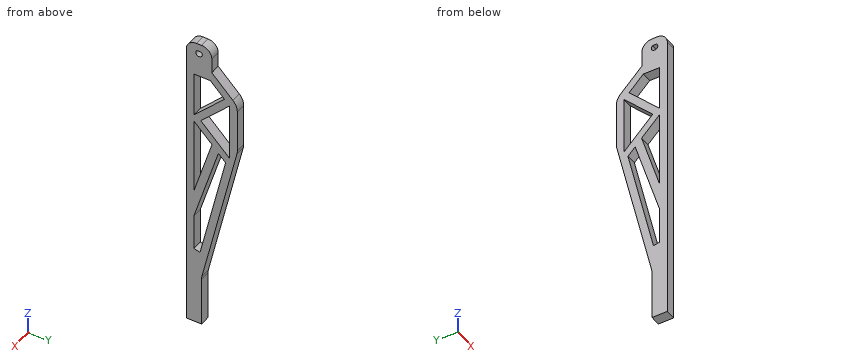
from build123d import *

# Parameters (mm, degrees)
BOSS_EXTRUDE1_DEPTH = 10
CUT_EXTRUDE2_DEPTH  = 305.302481094
FILLET1_R           = 10
FILLET2_R           = 15


with BuildPart() as part:
    # Sketch1 → Boss-Extrude1 (new body)
    with BuildSketch(Plane(origin=(0, 0, 0), x_dir=(0, 0, -1), z_dir=(1, 0, 0))):
        Polygon((0, 0), (300, 0), (300, 15), (250, 15), (100, 50), (50, 50), (25, 25), (0, 25), align=None)
    extrude(amount=-BOSS_EXTRUDE1_DEPTH)

    # Sketch2 → Cut-Extrude2 (cut, through all)
    with BuildSketch(Plane(origin=(0, 0, 0), x_dir=(0, 0, -1), z_dir=(1, 0, 0))):
        Polygon((53.106601718, 42.5), (109.675144213, 42.5), (81.390872965, 14.215728753), align=None)
        Polygon((34.106601718, 23.5), (34.106601718, 7.5), (78.051863034, 7.5), (48.079232376, 37.472630658), align=None)
        Polygon((102.407552426, 25.17766953), (84.729882897, 7.5), (159.744277132, 7.5), align=None)
        Polygon((116.052511988, 38.552952969), (223.422310427, 13.5), (222.022310427, 7.5), (186.765608253, 7.5), (108.981444176, 31.481885157), align=None)
        with BuildLine():
            Line((7.46, 14.446381258), (7.46, 10.553618742))
            ThreePointArc((7.46, 10.553618742), (13.2, 12.5), (7.46, 14.446381258))
        make_face()
    extrude(amount=-CUT_EXTRUDE2_DEPTH, mode=Mode.SUBTRACT)

    # Fillet1
    fillet1_edges = [part.edges().sort_by_distance(p)[0] for p in [
        (-5, 25, 0),
        (-5, 0, 0),
    ]]
    fillet(fillet1_edges, radius=FILLET1_R)

    # Fillet2
    fillet2_edges = [part.edges().sort_by_distance(p)[0] for p in [
        (-5, 50, -50),
        (-5, 50, -100),
        (-5, 15, -250),
    ]]
    fillet(fillet2_edges, radius=FILLET2_R)


solid = part.part
Check sheet for the modelled part. Datum: model origin and axes. Units: mm. Round coordinates to 2 decimals unless told otherwise and drop trailing zeros. Order: outer loops, then holes, each group sorted by start corner. A loop starts at its lowest first (then second) coordinate and runs counter-clockwise, first axis right, second up.
(1) Cross-section at B-B, the plane x = -5.25. State how many separate pieces and enclosed holes the cut face has, and give its area (3 significant figures).
(2) Cross-section at A-A, the plane z = -65. Enter the section's corners in (x, y), and give its area (3 significant figures).
(3) Scan lines: probe 1 along Y at (x, z) = (-3, -107); probe 2 along Y at (x, z) = (-3.25, -115.5); probe 3 along Y at (x, z) = (-9, -283). Record each from-to range of solid material in increasing order.
(4) Cross-section at D-D, the plane z = -181. Enter the section's corners in (x, y).
(5) Cross-section at C-C, the plane y = 21. Enter the section's corners in (x, z).
(6) Go/stop test with flat-tipped pins: P1, Ø4, axis at x = -6, y = 21, coming from the +Z side; P2, Ø5, axis at x = -6.5, z = -120, coming from the +Y side; P3, Ø3, axis at x = -6, z = -210, coming from the +Y side. Record where each tip stops, or that it passes through.
Check sheet entries:
1. separate pieces: 1
1. enclosed holes: 5
1. area: 6,130 mm2
2. outline: (-10, 0) - (0, 0) - (0, 7.5) - (-10, 7.5) - close; (-10, 20.55) - (0, 20.55) - (0, 30.61) - (-10, 30.61) - close; (-10, 42.5) - (0, 42.5) - (0, 50) - (-10, 50) - close
2. area: 251 mm2
3. probe 1: y = 0 to 7.5, 23.76 to 39.82, 42.5 to 48.37
3. probe 2: y = 0 to 7.5, 21.14 to 29.47, 38 to 46.38
3. probe 3: y = 0 to 15
4. outline: (-10, 0) - (0, 0) - (0, 9.28) - (-10, 9.28) - close; (-10, 23.4) - (0, 23.4) - (0, 31.1) - (-10, 31.1) - close
5. outline: (-10, -224.29) - (0, -224.29) - (0, -191.28) - (-10, -191.28) - close; (-10, -142.98) - (0, -142.98) - (0, -115.96) - (-10, -115.96) - close; (-10, -98.23) - (0, -98.23) - (0, -88.18) - (-10, -88.18) - close; (-10, -74.61) - (0, -74.61) - (0, -64.55) - (-10, -64.55) - close; (-10, -34.11) - (0, -34.11) - (0, -2) - (-10, -2) - close
6. P1: stops at z = -0.83
6. P2: stops at y = 45.92
6. P3: stops at y = 24.68
